Autodesk Inventor part; units mm, degrees
ref_plane "YZ Plane" through (0, 0, 0) normal (1, 0, 0) x (0, 1, 0)
ref_plane "XZ Plane" through (0, 0, 0) normal (0, 1, 0) x (-1, 0, 0)
ref_plane "XY Plane" through (0, 0, 0) normal (0, 0, 1) x (1, 0, 0)
sketch "Sketch1" plane through (0, 0, 0) normal (0, 0, 1) x (1, 0, 0)
  line L0 (36.83, -35.56) -> (-36.83, -35.56) construction
  line L1 (-36.83, -35.56) -> (-36.83, 35.56) construction
  line L2 (-36.83, 35.56) -> (36.83, 35.56) construction
  line L3 (36.83, 35.56) -> (36.83, -35.56) construction
  line L4 (36.83, -35.56) -> (-36.83, 35.56) construction
  line L5 (-36.83, -35.56) -> (36.83, 35.56) construction
  arc A0 (-31.75, 35.56) -> (-36.83, 30.48) centre (-31.75, 30.48) ccw construction
  arc A1 (36.83, 30.48) -> (31.75, 35.56) centre (31.75, 30.48) ccw construction
  arc A2 (-36.83, -30.48) -> (-31.75, -35.56) centre (-31.75, -30.48) ccw construction
  arc A3 (31.75, -35.56) -> (36.83, -30.48) centre (31.75, -30.48) ccw construction
  line L6 (31.75, -35.687) -> (-31.75, -35.687)
  line L7 (-36.957, -30.48) -> (-36.957, 30.48)
  line L8 (-31.75, 35.687) -> (31.75, 35.687)
  line L9 (36.957, 30.48) -> (36.957, -30.48)
  line L10 (36.957, -35.687) -> (-36.957, 35.687) construction
  line L11 (-36.957, -35.687) -> (36.957, 35.687) construction
  arc A4 (36.957, 30.48) -> (31.75, 35.687) centre (31.75, 30.48) ccw
  arc A5 (-31.75, 35.687) -> (-36.957, 30.48) centre (-31.75, 30.48) ccw
  arc A6 (-36.957, -30.48) -> (-31.75, -35.687) centre (-31.75, -30.48) ccw
  arc A7 (31.75, -35.687) -> (36.957, -30.48) centre (31.75, -30.48) ccw
  line L12 (-31.75, 36.887) -> (31.75, 36.887)
  line L13 (38.157, 30.48) -> (38.157, -30.48)
  line L14 (-31.75, -36.887) -> (31.75, -36.887)
  line L15 (-38.157, -30.48) -> (-38.157, 30.48)
  arc A8 (-31.75, 36.887) -> (-38.157, 30.48) centre (-31.75, 30.48) ccw
  arc A9 (38.157, 30.48) -> (31.75, 36.887) centre (31.75, 30.48) ccw
  arc A10 (31.75, -36.887) -> (38.157, -30.48) centre (31.75, -30.48) ccw
  arc A11 (-38.157, -30.48) -> (-31.75, -36.887) centre (-31.75, -30.48) ccw
  line L16 (-36.957, 25.4) -> (-31.75, 25.4)
  line L17 (-26.67, 35.687) -> (-26.67, 30.48)
  arc A12 (-31.75, 25.4) -> (-26.67, 30.48) centre (-31.75, 30.48) ccw
  circle A13 centre (-31.75, 30.48) radius 1.7145
  line L18 (0, 0) -> (78.9567, 0) construction
  line L19 (0, 0) -> (0, 57.9461) construction
  line L20 (36.957, 25.4) -> (31.75, 25.4)
  line L21 (26.67, 35.687) -> (26.67, 30.48)
  arc A14 (26.67, 30.48) -> (31.75, 25.4) centre (31.75, 30.48) ccw
  circle A15 centre (31.75, 30.48) radius 1.7145
  line L22 (-36.957, -25.4) -> (-31.75, -25.4)
  line L23 (-26.67, -35.687) -> (-26.67, -30.48)
  arc A16 (-26.67, -30.48) -> (-31.75, -25.4) centre (-31.75, -30.48) ccw
  circle A17 centre (-31.75, -30.48) radius 1.7145
  line L24 (36.957, -25.4) -> (31.75, -25.4)
  arc A18 (31.75, -25.4) -> (26.67, -30.48) centre (31.75, -30.48) ccw
  line L25 (26.67, -35.687) -> (26.67, -30.48)
  circle A19 centre (31.75, -30.48) radius 1.7145
  dimension "d0" = 73.66
  dimension "d1" = 71.12
  dimension "d2" = 5.08
  dimension "d4" = 0.127
  dimension "d5" = 0.127
  dimension "d7" = 1.2
  dimension "d12" = 10.16
  dimension "d13" = 10.16
  dimension "d14" = 3.429
  dimension "d22" = 1.2
extrude "Extrusion1" add sketch "Sketch1" along normal blind 5.08 contours L12 A9 L13 A10 L14 A11 L15 A8
extrude "Extrusion2" add sketch "Sketch1" along normal blind 3.302 contours L6 L25 A18 L24 L9 A7 | L6 A6 L7 L22 A16 L23 | L20 A14 L21 L8 A4 L9 | L7 A5 L8 L17 A12 L16
sketch "Sketch2" plane through (-38.157, -30.48, 0) normal (-1, 0, 0) x (0, 0, 1)
  line L0 (0, 0) -> (0, -6.407)
  line L1 (0, -6.407) -> (5.08, -6.407)
  line L2 (5.08, 0) -> (5.08, -6.407)
  line L3 (0, 0) -> (5.08, 0)
  line L4 (0, 60.96) -> (0, 0)
  line L5 (0, 0) -> (5.08, 0)
  line L6 (5.08, 60.96) -> (5.08, 0)
  line L7 (0, 60.96) -> (5.08, 60.96)
  line L8 (0, 67.367) -> (0, 60.96)
  line L9 (0, 60.96) -> (5.08, 60.96)
  line L10 (5.08, 67.367) -> (5.08, 60.96)
  line L11 (0, 67.367) -> (5.08, 67.367)
  line L12 (-16.8443, 22.549) -> (26.7617, 22.549) construction
  line L13 (5.08, 0) -> (5.08, 60.96) construction
  line L14 (2.032, 28.899) -> (5.08, 28.899)
  line L15 (5.08, 28.899) -> (5.08, 16.199) construction
  line L16 (5.08, 16.199) -> (2.032, 16.199)
  line L17 (2.032, 16.199) -> (2.032, 28.899)
  line L18 (2.032, 28.899) -> (5.08, 16.199) construction
  line L19 (5.08, 28.899) -> (2.032, 16.199) construction
  point P0 (0, 30.48)
  point P1 (3.556, 22.549)
  dimension "d17" = 28.956
  dimension "d18" = 12.7
  dimension "d19" = 3.048
extrude "Extrusion3" cut sketch "Sketch2" against normal blind 2.54 contours L16 L17 L14 L6
properties part number "bumper"
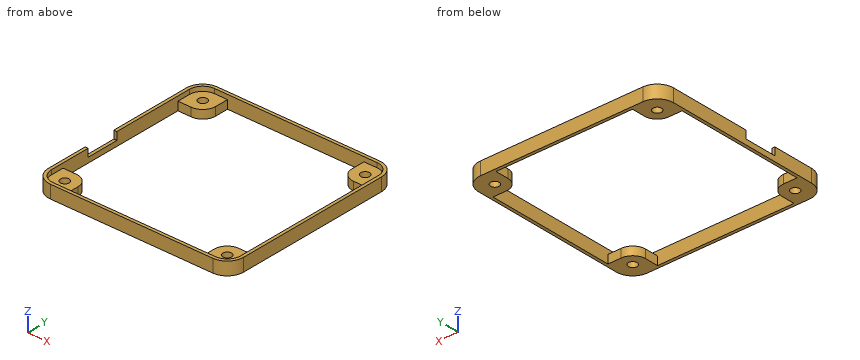
Model file for the job. Use its own axes, mm. Give positions to 0.01 mm unless a question says otherwise; leave off trailing zeros. Loops run counter-clockwise (first coordinate to the right, second up) from the corner with the lowest first, then second, coordinate; pieces in that order, holes last.
Item 1: Slice it at A-A (y = -3). Write the cut outline in (x, z).
Check values:
outline: (-38.16, 0) - (-36.96, 0) - (-36.96, 2.03) - (-38.16, 2.03) - close; (36.96, 0) - (38.16, 0) - (38.16, 5.08) - (36.96, 5.08) - close
Item 2: Drop flat-ended pins along their axis: P1, Ø1, axis at x = -38, y = -6, coming from the +Z side; P2, Ø2.5, axis at x = 33.5, z = 1.5, coming from the +Y side; P3, Ø0.6, axis at x = -37.5, z = 3.5, coming from the -Y side. Give the stop position or say it passes through.
Check values:
P1: stops at z = 2.03
P2: stops at y = 36.87
P3: stops at y = -33.85
Item 3: Slice it at C-C (x = 3.5). Write the cut outline in (y, z).
Check values:
outline: (-36.89, 0) - (-35.69, 0) - (-35.69, 5.08) - (-36.89, 5.08) - close; (35.69, 0) - (36.89, 0) - (36.89, 5.08) - (35.69, 5.08) - close
Item 4: Drill centre lines: line 1 along Y through (x, z) = (-31.75, 0.85); line 2 along Y through (x, z) = (23, 4.9); line 3 along X through (y, z) = (23.5, 3.25). Where is each one in solid material? Low to high.
Check values:
line 1: y = -36.89 to -32.19, -28.77 to -25.4, 25.4 to 28.77, 32.19 to 36.89
line 2: y = -36.89 to -35.69, 35.69 to 36.89
line 3: x = -38.16 to -36.96, 36.96 to 38.16
Item 5: Slice it at B-B (z = 1.05). Write the cut outline in (x, y).
Check values:
outline: (-38.16, -30.48) arc R6.41 ccw to (-31.75, -36.89) - (31.75, -36.89) arc R6.41 ccw to (38.16, -30.48) - (38.16, 30.48) arc R6.41 ccw to (31.75, 36.89) - (-31.75, 36.89) arc R6.41 ccw to (-38.16, 30.48) - close; hole (-36.96, -25.4) - (-31.75, -25.4) arc R5.08 cw to (-26.67, -30.48) - (-26.67, -35.69) - (26.67, -35.69) - (26.67, -30.48) arc R5.08 cw to (31.75, -25.4) - (36.96, -25.4) - (36.96, 25.4) - (31.75, 25.4) arc R5.08 cw to (26.67, 30.48) - (26.67, 35.69) - (-26.67, 35.69) - (-26.67, 30.48) arc R5.08 cw to (-31.75, 25.4) - (-36.96, 25.4) - close; hole circle Ø3.43 at (-31.75, -30.48); hole circle Ø3.43 at (-31.75, 30.48); hole circle Ø3.43 at (31.75, -30.48); hole circle Ø3.43 at (31.75, 30.48)
Item 6: Slice it at D-D (x = -28). Write the cut outline in (y, z).
Check values:
outline: (-36.89, 0) - (-27.05, 0) - (-27.05, 3.3) - (-35.69, 3.3) - (-35.69, 5.08) - (-36.89, 5.08) - close; (27.05, 0) - (36.89, 0) - (36.89, 5.08) - (35.69, 5.08) - (35.69, 3.3) - (27.05, 3.3) - close
